For this review, take the finished solid that the model builds, in its own axes (mm). Face numbers are marked on the shaded views. A direction names the side the tool comes from. Coordinates: 2 decimals unless noted, no trailing zeros. Order: outer loops, then holes, each group sorted by start corner. A loop starts at its lowest first (then second) coordinate and runs counter-clockwise, first axis right, second up. Notation, with made-up numbers: (77.5, -12.5) -> (123.5, -12.5) arc R17 cw to (123.5, -4.5) -> close; hole circle Ø10 at (89.25, 11). An arc over 180 degrees is marked (long way). Write item = value, one per line. Start each with the question number.
1) Consider section D-D on y = -12. Give the boundary of the cut face in (x, z).
2) Wall thickness on probe 1 along X at (y, z) = (-2, -19); probe 2 along Z at (x, y) = (-12, -22); probe 3 along Y at (x, z) = (6, -17): over which ranges is each line inside the solid? List them lowest first. Write a range as [from, to].
3) Consider section A-A on z = -21.5. Give the boundary of the cut face in (x, y), and give its area (3 significant figures).
4) Machinability: for the marked faces 1, 2, 3, 4 and 5, which of the approach directions +Z, -Z, +X, -X, +Y, -Y give a long, thin tool a straight path to every point of the face, cutting with its end or side? Answer none if there is none.
5) Insertion check: pin 1 Ø13 at (x, z) = (-7, -19) entering from +Y; pin 2 Ø7 at (y, z) = (12.5, -16) entering from +X; pin 3 Ø5.5 at (x, y) = (5.5, -19.5) entering from -Z. Each pin has a flat end and moves straight along its axis. Give the tip position at first contact, or say it passes through.
6) Consider section C-C on x = 0. Give the boundary of the cut face in (y, z).
7) Consider section B-B on x = -9.25. Give the boundary of the cut face in (y, z).
from build123d import *

# Parameters (mm, degrees)
SKIZZE1_W                                            = 50.5
SKIZZE1_H                                            = 50.5
AUFSATZ_LINEAR_AUSTRAGEN1_DEPTH                      = 6.1
AUFSATZ_LINEAR_AUSTRAGEN2_DEPTH                      = 3
SKIZZE3_R                                            = 21.4
AUFSATZ_LINEAR_AUSTRAGEN3_DEPTH                      = 12
SKIZZE4_W                                            = 31.8
SKIZZE4_H                                            = 24
AUFSATZ_LINEAR_AUSTRAGEN4_DEPTH                      = 16
FORMSENKUNG_F_R_M3_LINSENSENKSCHRAUBE_MI_D           = 3.4
FORMSENKUNG_F_R_M3_LINSENSENKSCHRAUBE_MI_CSINK_D     = 6.3
FORMSENKUNG_F_R_M3_LINSENSENKSCHRAUBE_MI_CSINK_ANGLE = 90
VERRUNDUNG1_R                                        = 3
SKIZZE7_R                                            = 19.5
SCHNITT_LINEAR_AUSTRAGEN1_DEPTH                      = 18
F_4_4_4_4_DURCHMESSER_BOHRUNG1_D                     = 4.4
SKIZZE10_W                                           = 10.3
SKIZZE10_H                                           = 6.423058333
AUFSATZ_LINEAR_AUSTRAGEN5_DEPTH                      = 6.3


with BuildPart() as part:
    # Skizze1 → Aufsatz-Linear austragen1 (new body)
    with BuildSketch(Plane.XY):
        Rectangle(SKIZZE1_W, SKIZZE1_H)
    extrude(amount=AUFSATZ_LINEAR_AUSTRAGEN1_DEPTH)

    # Skizze2 → Aufsatz-Linear austragen2 (add)
    with BuildSketch(Plane.XY.offset(6.1)):
        with BuildLine():
            Line((-4.5, -21.023796042), (-4.5, 21.023796042))
            ThreePointArc((-4.5, 21.023796042), (-21.5, 0), (-4.5, -21.023796042))
        make_face()
        with BuildLine():
            ThreePointArc((4.5, 21.023796042), (0, 21.5), (-4.5, 21.023796042))
            Line((-4.5, 21.023796042), (-4.5, -21.023796042))
            ThreePointArc((-4.5, -21.023796042), (0, -21.5), (4.5, -21.023796042))
            Line((4.5, -21.023796042), (4.5, 21.023796042))
        make_face()
        with BuildLine():
            ThreePointArc((21.5, 0), (16.718253497, 13.518505835), (4.5, 21.023796042))
            Line((4.5, 21.023796042), (4.5, -21.023796042))
            ThreePointArc((4.5, -21.023796042), (16.718253497, -13.518505835), (21.5, 0))
        make_face()
        with BuildLine():
            Line((4.5, 23.4), (-4.5, 23.4))
            Line((-4.5, 23.4), (-4.5, 21.023796042))
            ThreePointArc((-4.5, 21.023796042), (0, 21.5), (4.5, 21.023796042))
            Line((4.5, 21.023796042), (4.5, 23.4))
        make_face()
        with BuildLine():
            ThreePointArc((4.5, -21.023796042), (0, -21.5), (-4.5, -21.023796042))
            Line((-4.5, -21.023796042), (-4.5, -23.4))
            Line((-4.5, -23.4), (4.5, -23.4))
            Line((4.5, -23.4), (4.5, -21.023796042))
        make_face()
    extrude(amount=AUFSATZ_LINEAR_AUSTRAGEN2_DEPTH)

    # Skizze3 → Aufsatz-Linear austragen3 (add)
    with BuildSketch(Plane(origin=(0, 0, 0), x_dir=(-1, 0, 0), z_dir=(0, 0, -1))):
        Circle(SKIZZE3_R)
    extrude(amount=AUFSATZ_LINEAR_AUSTRAGEN3_DEPTH)

    # Skizze4 → Aufsatz-Linear austragen4 (add)
    with BuildSketch(Plane(origin=(0, 0, -12), x_dir=(-1, 0, 0), z_dir=(0, 0, -1))):
        with Locations((0, -2.323058333)):
            Rectangle(SKIZZE4_W, SKIZZE4_H)
    extrude(amount=AUFSATZ_LINEAR_AUSTRAGEN4_DEPTH)

    # Formsenkung für M3 Linsensenkschraube mit Schlitz1 (through all)
    with Locations(Plane.XY.offset(6.1)):
        with Locations((-19, 19), (19, 19), (19, -19), (-19, -19)):
            CounterSinkHole(FORMSENKUNG_F_R_M3_LINSENSENKSCHRAUBE_MI_D / 2, FORMSENKUNG_F_R_M3_LINSENSENKSCHRAUBE_MI_CSINK_D / 2, counter_sink_angle=FORMSENKUNG_F_R_M3_LINSENSENKSCHRAUBE_MI_CSINK_ANGLE)

    # Verrundung1
    verrundung1_edges = [part.edges().sort_by_distance(p)[0] for p in [
        (25.25, -25.25, 3.05),
        (-25.25, -25.25, 3.05),
        (-25.25, 25.25, 3.05),
        (25.25, 25.25, 3.05),
    ]]
    fillet(verrundung1_edges, radius=VERRUNDUNG1_R)

    # Skizze7 → Schnitt-Linear austragen1 (cut)
    with BuildSketch(Plane.XY.offset(9.1)):
        Circle(SKIZZE7_R)
    extrude(amount=-SCHNITT_LINEAR_AUSTRAGEN1_DEPTH, mode=Mode.SUBTRACT)

    # Ø4.4 (4.4) Durchmesser Bohrung1 (through all)
    with Locations(Plane.XY.offset(-8.9)):
        with Locations((-9.25, 0), (9.25, 0)):
            Hole(F_4_4_4_4_DURCHMESSER_BOHRUNG1_D / 2)

    # Skizze10 → Aufsatz-Linear austragen5 (add)
    with BuildSketch(Plane(origin=(0, 0, -12), x_dir=(-1, 0, 0), z_dir=(0, 0, -1))):
        with Locations((0, 12.888470834)):
            Rectangle(SKIZZE10_W, SKIZZE10_H)
    extrude(amount=AUFSATZ_LINEAR_AUSTRAGEN5_DEPTH)


solid = part.part
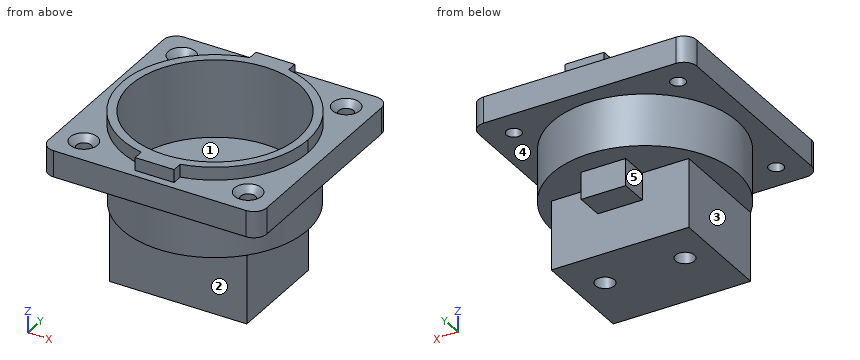
Answer sheet:
q1.outline = (-25.25, 0) -> (-17.72, 0) -> (-17.72, -12) -> (-15.9, -12) -> (-15.9, -28) -> (15.9, -28) -> (15.9, -12) -> (17.72, -12) -> (17.72, 0) -> (25.25, 0) -> (25.25, 6.1) -> (17.84, 6.1) -> (17.84, 9.1) -> (15.37, 9.1) -> (15.37, -8.9) -> (-15.37, -8.9) -> (-15.37, 9.1) -> (-17.84, 9.1) -> (-17.84, 6.1) -> (-25.25, 6.1) -> close
q2.probe_1 = [-15.9, -10.17], [-8.33, 8.33], [10.17, 15.9]
q2.probe_2 = [0, 6.1]
q2.probe_3 = [-14.32, 9.68]
q3.outline = (-15.9, -14.32) -> (15.9, -14.32) -> (15.9, 9.68) -> (-15.9, 9.68) -> close; hole circle Ø4.4 at (-9.25, 0); hole circle Ø4.4 at (9.25, 0)
q3.area = 733 mm2
q4.face_1 = +Z
q4.face_2 = -Z, +X, -X, -Y
q4.face_3 = -Z, -X, +Y, -Y
q4.face_4 = -Z
q4.face_5 = -Z, -X, +Y
q5.pin_1 = 16.1
q5.pin_2 = 15.9
q5.pin_3 = -12
q6.outline = (-25.25, 0) -> (-21.4, 0) -> (-21.4, -12) -> (-14.32, -12) -> (-14.32, -28) -> (9.68, -28) -> (9.68, -18.3) -> (16.1, -18.3) -> (16.1, -12) -> (21.4, -12) -> (21.4, 0) -> (25.25, 0) -> (25.25, 6.1) -> (23.4, 6.1) -> (23.4, 9.1) -> (19.5, 9.1) -> (19.5, -8.9) -> (-19.5, -8.9) -> (-19.5, 9.1) -> (-23.4, 9.1) -> (-23.4, 6.1) -> (-25.25, 6.1) -> close
q7.outline = (-25.25, 0) -> (-19.3, 0) -> (-19.3, -12) -> (-14.32, -12) -> (-14.32, -28) -> (-2.2, -28) -> (-2.2, -8.9) -> (-17.17, -8.9) -> (-17.17, 9.1) -> (-19.41, 9.1) -> (-19.41, 6.1) -> (-25.25, 6.1) -> close; (2.2, -28) -> (9.68, -28) -> (9.68, -12) -> (19.3, -12) -> (19.3, 0) -> (25.25, 0) -> (25.25, 6.1) -> (19.41, 6.1) -> (19.41, 9.1) -> (17.17, 9.1) -> (17.17, -8.9) -> (2.2, -8.9) -> close
